For this review, take the finished solid that the model builds, in its own axes (mm). A direction names the side the tool comes from. Round coordinates to 2 decimals unless told otherwise and drop trailing zeros. Write each loop counter-clockwise with the first axis right and the second up, starting at its lowest first coordinate (ties: lowest second). Pieces come first, ordered by that corner, then holes. Notation, with made-up numbers: (46.25, 56) -> (62.25, 56) arc R23 ccw to (62.25, 76) -> close; hole circle Ø1 at (-29, 40). An arc over 180 degrees is marked (long way). Answer in a Markdown table with one row per item. Add a question column.
```python
from build123d import *

# Parameters (mm, degrees)
F1_R     = 22.343097
F1_W     = 16.999803
F1_H     = 12.462489
F1_R_2   = 12.978797
F2_DEPTH = 88.24669


with BuildPart() as f2:
    # F1 (on offset) → F2 (new body)
    with BuildSketch(Plane.XY.offset(152.4)):
        with BuildLine():
            Line((43.658363, -9.476985), (44.675116, 0))
            ThreePointArc((44.675116, 0), (0, 44.675116), (-44.675116, 0))
            Line((-44.675116, 0), (-43.636028, -9.579299))
            ThreePointArc((-43.636028, -9.579299), (0.052362, -44.675085), (43.658363, -9.476985))
        make_face()
        Circle(F1_R, mode=Mode.SUBTRACT)
        with BuildLine():
            ThreePointArc((43.658363, -9.476985), (44.4202, -4.765685), (44.675116, 0))
            Line((44.675116, 0), (43.658363, -9.476985))
        make_face()
        with BuildLine():
            Line((-43.636028, -9.579299), (-44.675116, 0))
            ThreePointArc((-44.675116, 0), (-44.414584, -4.817745), (-43.636028, -9.579299))
        make_face()
        with BuildLine():
            Line((31.697058, -120.966422), (43.658363, -9.476985))
            ThreePointArc((43.658363, -9.476985), (0.052362, -44.675085), (-43.636028, -9.579299))
            Line((-43.636028, -9.579299), (-31.876086, -117.9937))
            ThreePointArc((-31.876086, -117.9937), (-0.213975, -85.687518), (31.878959, -117.565759))
            ThreePointArc((31.878959, -117.565759), (31.833451, -119.268521), (31.697058, -120.966422))
        make_face()
        with Locations((8.499901, -70.339483)):
            Rectangle(F1_W, F1_H, mode=Mode.SUBTRACT)
        with BuildLine():
            ThreePointArc((-31.226448, -123.982685), (1.526377, -149.408154), (31.697058, -120.966422))
            ThreePointArc((31.697058, -120.966422), (31.833451, -119.268521), (31.878959, -117.565759))
            ThreePointArc((31.878959, -117.565759), (-0.213975, -85.687518), (-31.876086, -117.9937))
            Line((-31.876086, -117.9937), (-31.226448, -123.982685))
        make_face()
        with Locations((0, -117.565759)):
            Circle(F1_R_2, mode=Mode.SUBTRACT)
        with BuildLine():
            Line((-31.226448, -123.982685), (-31.876086, -117.9937))
            ThreePointArc((-31.876086, -117.9937), (-31.69305, -121.003572), (-31.226448, -123.982685))
        make_face()
    extrude(amount=F2_DEPTH)


solid = f2.part
```
1. We need section B-B (x = 20). Write out the cut boundary in (y, z).
2. We need section C-C (y = 20). Write out the cut boundary in (x, z).
3. We need section D-D (x = -39). Write out the cut boundary in (y, z), plus the area to 3 significant figures.
4. For L1, parallel to Y at x = 3, z = 225; L2, parallel to Y at x = -9, z = 216; L3, parallel to X at y = -1, z = 182.5, list the stretches that pass through material, from the lowest coordinate up. Write a range as [from, to].
5. Tool access review of faces 1 (the flat face through (8, -64.108, 196)), 2 (the cylindrical face through (-31.698, -120.962, 195.906)): name each direction out of +Z, -Z, +X, -X, +Y, -Y from which nothing blocks a thin tool from reaching the whole face with its end or side.
6. The part is to be moulded in two halves that separate along Y. For faces 3 (the flat face through (0, -70, 196)), 4 (the flat face through (37.594, -66.002, 195.906)), 5 (the flat face through (-1, -51, 240.647)), say which applies: pulls with the +Y half, pulls with the -Y half, needs draft (parallel to the pull), parting line crosses it, or undercut.
7. We need section A-A (z = 166.5). Write out the cut boundary in (x, y).
8. Clearance check with flat-ended pins moving along their axes: pin 1 Ø18.5 at (x, z) = (8, 186) entering from -Y; pin 2 Ø1 at (y, z) = (-118, 166.5) entering from -X; pin 3 Ø2 at (y, z) = (-109.5, 203) entering from +X; pin 4 Ø1.5 at (x, z) = (-12, 209) entering from +Y. State where each tip first meets the part, or that it passes through.
Response:
| question | item | result |
|---|---|---|
| 1 | outline | (-142.39, 152.4) -> (-9.96, 152.4) -> (-9.96, 240.65) -> (-142.39, 240.65) -> close; (9.96, 152.4) -> (39.95, 152.4) -> (39.95, 240.65) -> (9.96, 240.65) -> close |
| 2 | outline | (-39.95, 152.4) -> (-9.96, 152.4) -> (-9.96, 240.65) -> (-39.95, 240.65) -> close; (9.96, 152.4) -> (39.95, 152.4) -> (39.95, 240.65) -> (9.96, 240.65) -> close |
| 3 | outline | (-52.32, 152.4) -> (21.79, 152.4) -> (21.79, 240.65) -> (-52.32, 240.65) -> close |
| 3 | area | 6,540 mm2 |
| 4 | L1 | [-149.3, -130.19], [-104.94, -76.57], [-64.11, -22.14], [22.14, 44.57] |
| 4 | L2 | [-148.15, -126.92], [-108.21, -20.45], [20.45, 43.76] |
| 4 | L3 | [-44.66, -22.32], [22.32, 44.66] |
| 5 | face 1 | +Z, -Z |
| 5 | face 2 | +Z, -Z, -X, -Y |
| 6 | face 3 | undercut |
| 6 | face 4 | pulls with the -Y half |
| 6 | face 5 | needs draft |
| 7 | outline | (-44.68, 0) arc R44.68 ccw to (-43.64, -9.58) -> (-31.88, -117.99) arc R31.88 ccw to (-31.23, -123.98) arc R31.88 ccw to (31.7, -120.97) -> (43.66, -9.48) arc R44.68 ccw to (44.68, 0) arc R44.68 ccw to start; hole circle Ø44.69 at (0, 0); hole circle Ø25.96 at (0, -117.57); hole (0, -76.57) -> (17, -76.57) -> (17, -64.11) -> (0, -64.11) -> close |
| 8 | pin 1 | y = -149.44 |
| 8 | pin 2 | x = -31.93 |
| 8 | pin 3 | x = 33.03 |
| 8 | pin 4 | y = 43.24 |
